CAD build for the part. Positions are in the model's coordinates, mm. Coordinates: 2 decimals unless noted, no trailing zeros. Write each loop counter-clockwise with the first axis right and the second up, starting at its lowest first coordinate (ties: lowest second). Pieces come first, ordered by that corner, then holes.
```python
from build123d import *

# Parameters (mm, degrees)
SKETCH1_R           = 1.5
BOSS_EXTRUDE1_DEPTH = 30
FILLET1_R           = 1.5
SCALE1_SCALE        = 2


with BuildPart() as part:
    # Sketch1 → Boss-Extrude1 (new body)
    with BuildSketch(Plane.XY):
        Circle(SKETCH1_R)
    extrude(amount=BOSS_EXTRUDE1_DEPTH)

    # Fillet1
    fillet1_edges = [part.edges().sort_by_distance(p)[0] for p in [
        (-1.5, 0, 0),
        (-1.5, 0, 30),
    ]]
    fillet(fillet1_edges, radius=FILLET1_R)


with BuildPart() as part_1:
    # Scale1: scaled about (0, 0, 15)
    add(part.part.scale(SCALE1_SCALE).moved(Location((0, 0, -15))))


solid = part_1.part
```
Item 1: Saw through at A-A, the plane y = 0. Write the cut outline in (x, z).
Item 2: Wall check: line 1 along Z through (x, y) = (-0.15, 0.15); line 2 along X through (y, z) = (0.1, 32); line 3 along Z through (x, y) = (-2.3, 1.4). Give the ranges that are in metal, low to high.
Item 3: Saw through at B-B, the plane z = -9. Write the cut outline in (x, y).
Working result:
1. outline: (-3, -12) arc R3 ccw to (3, -12) - (3, 42) arc R3 ccw to (-3, 42) - close
2. line 1: z = -14.99 to 44.99
2. line 2: x = -3 to 3
2. line 3: z = -13.32 to 43.32
3. outline: circle Ø6 at (0, 0)
